Input: part model. Units: mm. Frame: model coordinates. A direction names the side the tool comes from. Round coordinates to 2 decimals unless told otherwise and drop trailing zeros. Loops run counter-clockwise (first coordinate to the right, second up) from the corner with the lowest first, then second, coordinate; pieces in that order, holes last. Notation, with made-up numbers: (9.5, 29) - (40.5, 29) arc R4 cw to (40.5, 36) - close; hole circle Ø7 at (-27.75, 45.5). An arc over 180 degrees is marked (long way). Write each question's results on one line, items separated by ' | '.
from build123d import *

# Parameters (mm, degrees)
F1_DEPTH  = 30
F3_DEPTH  = 60
F4_R      = 7.5
F5_DEPTH  = 60.001
F6_W      = 40
F6_H      = 40
F7_DEPTH  = 30.001
F8_R      = 17
F9_DEPTH  = 13
F11_DEPTH = 10
F12_R     = 10
F13_DEPTH = 13.001


with BuildPart() as f1:
    # F0 (on Front) → F1 (new body)
    with BuildSketch(Plane.XZ):
        Polygon((0, 35), (0, 0), (60, 0), (60, 35), (50, 35), (50, 10), (10, 10), (10, 35), align=None)
    extrude(amount=F1_DEPTH)

    # F2 (on Right) → F3 (join)
    with BuildSketch(Plane.YZ):
        with BuildLine():
            Line((-30, 35), (0, 35))
            ThreePointArc((0, 35), (-15, 50), (-30, 35))
        make_face()
    extrude(amount=F3_DEPTH)

    # F4 (on face) → F5 (cut, through all)
    with BuildSketch(Plane.YZ.offset(60)):
        with Locations((-15, 35)):
            Circle(F4_R)
    extrude(amount=-F5_DEPTH, mode=Mode.SUBTRACT)

    # F6 (on Front) → F7 (cut, through all)
    with BuildSketch(Plane.XZ):
        with Locations((30, 30)):
            Rectangle(F6_W, F6_H)
    extrude(amount=F7_DEPTH, mode=Mode.SUBTRACT)

    # F8 (on face) → F9 (join)
    with BuildSketch(Plane.XY.offset(10)):
        with Locations((30, -15)):
            Circle(F8_R)
    extrude(amount=-F9_DEPTH)

    # F10 (on face) → F11 (join)
    with BuildSketch(Plane.XY.offset(10)):
        with BuildLine():
            Line((16, 0), (44, 0))
            ThreePointArc((44, 0), (30, 5.717143), (16, 0))
        make_face()
        with BuildLine():
            Line((44, -30), (16, -30))
            ThreePointArc((16, -30), (30, -35.717143), (44, -30))
        make_face()
    extrude(amount=-F11_DEPTH)

    # F12 (on face) → F13 (cut, through all)
    with BuildSketch(Plane.XY.offset(10)):
        with Locations((30, -14.282857)):
            Circle(F12_R)
    extrude(amount=-F13_DEPTH, mode=Mode.SUBTRACT)


solid = f1.part
1. Section query B-B, the plane y = -21. Output: boundary loops of the cut face in (x, z), plus the area to 3 significant figures.
Answer:
outline: (0, 0) - (14.09, 0) - (14.09, -3) - (22.59, -3) - (22.59, 10) - (10, 10) - (10, 30.5) - (0, 30.5) - close; (0, 39.5) - (10, 39.5) - (10, 48.75) - (0, 48.75) - close; (37.41, -3) - (45.91, -3) - (45.91, 0) - (60, 0) - (60, 30.5) - (50, 30.5) - (50, 10) - (37.41, 10) - close; (50, 39.5) - (60, 39.5) - (60, 48.75) - (50, 48.75) - close | area: 1,100 mm^2
2. Section query C-C, the plane z = 45. Output: boundary loops of the cut face in (x, y).
Answer:
outline: (0, -26.18) - (10, -26.18) - (10, -3.82) - (0, -3.82) - close; (50, -26.18) - (60, -26.18) - (60, -3.82) - (50, -3.82) - close
3. Contact query for flat-ended pins moving along their axis: pin 1 (12 mm diameter, centred on x = 36.5, y = -9.5, fed in from +Z); pin 2 (13 mm diameter, centred on x = 5.5, z = 17.5, fed in from +Y); pin 3 (12 mm diameter, centred on y = -15, z = 35, fed in from +X); pin 4 (8 mm diameter, centred on x = 55.5, z = 24, fed in from -Y). Output: stop coordinate, or through.
Answer:
pin 1: z = 10 | pin 2: y = 0 | pin 3: through | pin 4: y = -30
4. Set-up query: faces 1 (the flat face through (6, -30, 18)), 2 (the flat face through (30, -33, 0)), 3 (the flat face through (54, 0, 18)). Return all of +Z, -Z, +X, -X, +Y, -Y with unobstructed straight access to the full face (end or side cutting, diameter ignored); none if empty.
Answer:
face 1: +Z, -Z, -X, -Y | face 2: -Z | face 3: +Z, -Z, +X, +Y
5. Section query D-D, the plane x = 30. Output: boundary loops of the cut face in (y, z), plus the area to 3 significant figures.
Answer:
outline: (-35.72, 0) - (-32, 0) - (-32, -3) - (-24.28, -3) - (-24.28, 10) - (-35.72, 10) - close; (-4.28, -3) - (2, -3) - (2, 0) - (5.72, 0) - (5.72, 10) - (-4.28, 10) - close | area: 256 mm^2
6. Section query A-A, the plane x = 9. Output: boundary loops of the cut face in (y, z).
Answer:
outline: (-30, 0) - (0, 0) - (0, 35) arc R15 ccw to (-30, 35) - close; hole circle Ø15 at (-15, 35)
7. Mould query, pull axis Y, two halves, no side actions, for faces 4 (the flat face through (60, -15, 20)), 5 (the cylindrical face through (55.07, -16.63, 27.68)), 6 (the cylindrical face through (55, -15, 50)). Classes: pulls with the +Y half, pulls with the -Y half, needs draft (parallel to the pull), parting line crosses it, or undercut.
Answer:
face 4: needs draft | face 5: undercut | face 6: parting line crosses it
8. Line query: line 1 (Z direction, x = 52.75, y = -15); line 2 (X direction, y = -12, z = 42); line 3 (Y direction, x = 6, z = 35). Output: solid intervals per line, ascending. Write a range as [from, to].
Answer:
line 1: [0, 27.5], [42.5, 50] | line 2: [0, 10], [50, 60] | line 3: [-30, -22.5], [-7.5, 0]
